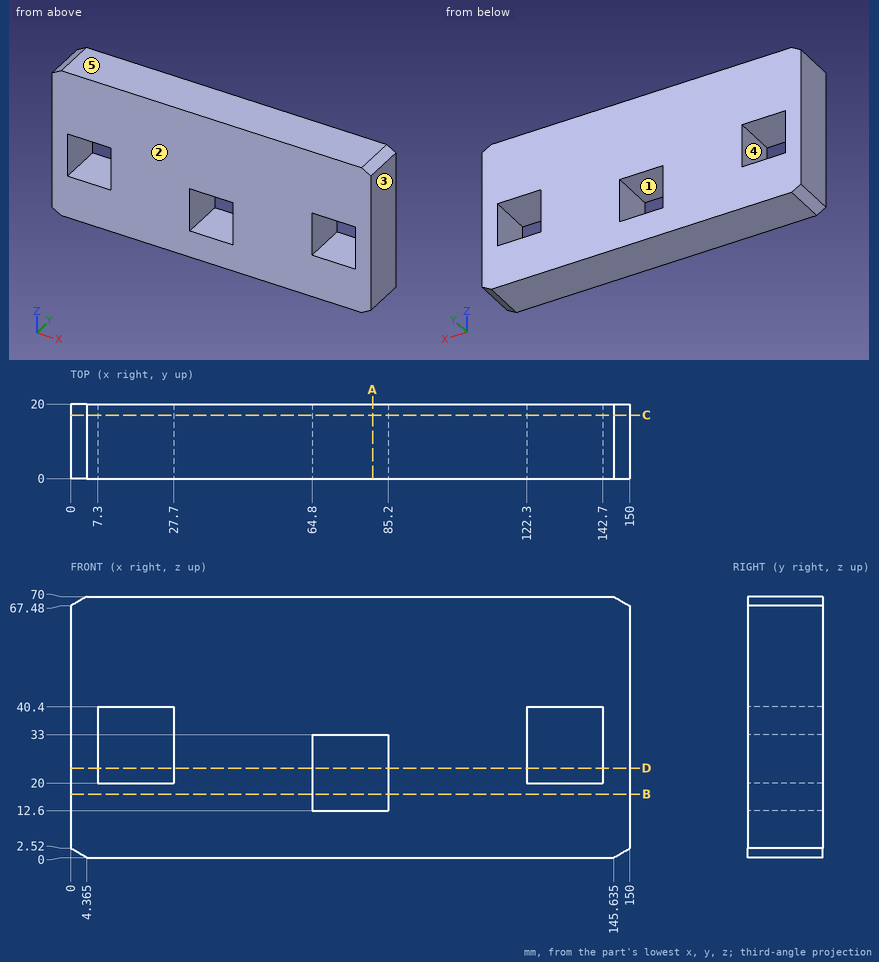
Design review of the part shown in the three views and the two pictorial views. Dimensions are in mm from the part's minimum x, y and z. A direction names the side the tool comes from. Give positions to 0.01 mm unless a question says otherwise; leave off trailing zeros. Write each loop counter-clockwise with the first axis right and the second up, starting at its lowest first coordinate (ties: lowest second). Pieces come first, ordered by that corner, then holes. Notation, with made-up numbers: M -38.5,15 L 4.5,15 A22 cw 4.5,34 Z; hole C 73.5,-3 d1. An arc over 180 degrees is marked long. Return JSON: item names as keys, results as strings. Group by question number.
Item 1: Tool access review of the marked faces 1 and 2: name each direction out of +Z, -Z, +X, -X, +Y, -Y from which nothing blocks a thin tool from reaching the whole face with its end or side.
Item 2: Take a section at A-A (x = 81). Give the boundary of the cut face in (y, z).
Item 3: Take a section at C-C (y = 17). Give the boundary of the cut face in (x, z) (1 decimal).
Item 4: Take a section at B-B (z = 17). Give the boundary of the cut face in (x, y), plus the area to 3 significant figures.
Item 5: The part is to be moulded in two halves that separate along X. For the marked faces 3, 4 and 5, say which applies: pulls with the +X half, pulls with the -X half, needs draft (parallel to the pull), parting line crosses it, or undercut.
Item 6: Wall thickness on line 1 along X through (y, z) = (2.5, 36); line 2 along X through (y, z) = (13.5, 24); line 3 along Z through (x, y) = (68.5, 18): over which ranges is each line inside the solid? List them lowest first.
Item 7: Take a section at D-D (z = 24). Give the boundary of the cut face in (x, y).
Return value:
{
 "1": {"face 1": "+Y, -Y", "face 2": "+Z, -Z, +X, -X, -Y"},
 "2": {"outline": "M 0,0 L 20,0 L 20,12.6 L 0,12.6 Z; M 0,33 L 20,33 L 20,70 L 0,70 Z"},
 "3": {"outline": "M 0,2.5 L 4.4,0 L 145.6,0 L 150,2.5 L 150,67.5 L 145.6,70 L 4.4,70 L 0,67.5 Z; hole M 7.3,20 L 27.7,20 L 27.7,40.4 L 7.3,40.4 Z; hole M 64.8,12.6 L 85.2,12.6 L 85.2,33 L 64.8,33 Z; hole M 122.3,20 L 142.7,20 L 142.7,40.4 L 122.3,40.4 Z"},
 "4": {"outline": "M 0,0 L 64.8,0 L 64.8,20 L 0,20 Z; M 85.2,0 L 150,0 L 150,20 L 85.2,20 Z", "area": "2,590 mm2"},
 "5": {"face 3": "pulls with the +X half", "face 4": "undercut", "face 5": "needs draft"},
 "6": {"line 1": "x = 0 to 7.3, 27.7 to 122.3, 142.7 to 150", "line 2": "x = 0 to 7.3, 27.7 to 64.8, 85.2 to 122.3, 142.7 to 150", "line 3": "z = 0 to 12.6, 33 to 70"},
 "7": {"outline": "M 0,0 L 7.3,0 L 7.3,20 L 0,20 Z; M 27.7,0 L 64.8,0 L 64.8,20 L 27.7,20 Z; M 85.2,0 L 122.3,0 L 122.3,20 L 85.2,20 Z; M 142.7,0 L 150,0 L 150,20 L 142.7,20 Z"}
}
